from build123d import *

# Parameters (mm, degrees)
SKETCH1_R                = 4.5
SKETCH1_R_2              = 2.5
BOSS_EXTRUDE1_DEPTH      = 0.5
SKETCH1_2_R              = 4.5
SKETCH1_2_R_2            = 2.5
BOSS_EXTRUDE2_DEPTH      = 18.5
BOSS_EXTRUDE2_DEPTH_BACK = 18.5


with BuildPart() as part:
    # Sketch1 → Boss-Extrude1 (new body, symmetric)
    with BuildSketch(Plane(origin=(0, 0, 0), x_dir=(1, 0, 0), z_dir=(0, 1, 0))):
        Circle(SKETCH1_R)
        Circle(SKETCH1_R_2, mode=Mode.SUBTRACT)
    extrude(amount=BOSS_EXTRUDE1_DEPTH, both=True)

    # Sketch1_2 → Boss-Extrude2 (add, two sides)
    with BuildSketch(Plane(origin=(0, 0, 0), x_dir=(1, 0, 0), z_dir=(0, 1, 0))) as boss_extrude2_sk:
        Circle(SKETCH1_2_R)
        Circle(SKETCH1_2_R_2, mode=Mode.SUBTRACT)
    extrude(amount=BOSS_EXTRUDE2_DEPTH)
    extrude(boss_extrude2_sk.sketch, amount=-BOSS_EXTRUDE2_DEPTH_BACK)


solid = part.part
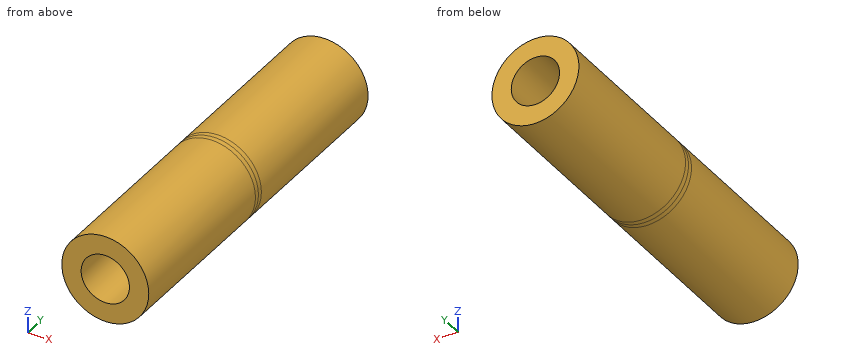
Can you work these out from the model? Positions are in its coordinate system, mm. Give positions to 0.01 mm unless a question says otherwise; leave off trailing zeros. Write each loop counter-clockwise with the first axis right and the second up, starting at its lowest first coordinate (ties: lowest second). Pieces come first, ordered by that corner, then holes. Notation, with made-up numbers: M 36.25,63.25 L 64.25,63.25 A6 cw 64.25,69.25 Z; hole C 72.25,63.5 d5. An arc over 180 degrees is marked long. Answer in a Markdown table with one row per item. Add a question column.
Item 1: Please list where these lines run through material, in increasing order: L1, parallel to X at y = 9.5, z = 0; L2, parallel to Z at x = -1, y = 2.5.
Item 2: Imagine slicing it at D-D, the plane x = -3.25. Write out the boundary of the cut face in (y, z).
Item 3: For pin 1 Ø4.5 at (x, z) = (0, 0) entering from +Y; pin 2 Ø1.5 at (y, z) = (0.5, 2) entering from +X; pin 3 Ø2 at (y, z) = (12.5, -2) entering from -X, each with a flat end and sliding along its axis, tell me the tip position at first contact or that it passes through.
Item 4: Imagine slicing it at B-B, the plane x = 0. Write out the boundary of the cut face in (y, z).
Item 5: Imagine slicing it at C-C, the plane y = 9.5. Write out the boundary of the cut face in (x, z), plus the area to 3 significant figures.
Item 6: Imagine slicing it at A-A, the plane z = 0. Write out the boundary of the cut face in (x, y), plus the area to 3 significant figures.
Evaluation:
| question | item | result |
|---|---|---|
| 1 | L1 | x = -4.5 to -2.5, 2.5 to 4.5 |
| 1 | L2 | z = -4.39 to -2.29, 2.29 to 4.39 |
| 2 | outline | M -18.5,-3.11 L 18.5,-3.11 L 18.5,3.11 L -18.5,3.11 Z |
| 3 | pin 1 | passes through |
| 3 | pin 2 | stops at x = 4.32 |
| 3 | pin 3 | stops at x = -4.39 |
| 4 | outline | M -18.5,-4.5 L 18.5,-4.5 L 18.5,-2.5 L -18.5,-2.5 Z; M -18.5,2.5 L 18.5,2.5 L 18.5,4.5 L -18.5,4.5 Z |
| 5 | outline | C 0,0 d9; hole C 0,0 d5 |
| 5 | area | 44.0 mm² |
| 6 | outline | M -4.5,-18.5 L -2.5,-18.5 L -2.5,18.5 L -4.5,18.5 Z; M 2.5,-18.5 L 4.5,-18.5 L 4.5,18.5 L 2.5,18.5 Z |
| 6 | area | 148 mm² |
